For this review, take the finished solid that the model builds, in its own axes (mm). Face numbers are marked on the shaded views. A direction names the side the tool comes from. Coordinates: 2 decimals unless noted, no trailing zeros. Order: outer loops, then holes, each group sorted by start corner. A loop starts at its lowest first (then second) coordinate and runs counter-clockwise, first axis right, second up.
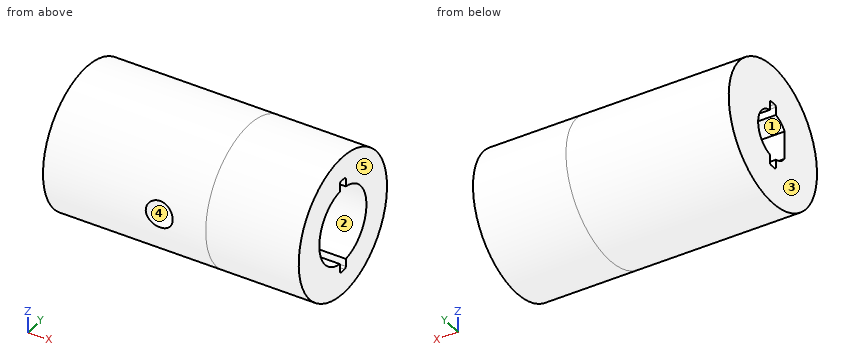
from build123d import *

# Parameters (mm, degrees)
SKETCH1_R            = 7.5
SKETCH1_R_2          = 4
SCREWSIDE_DEPTH      = 10
MOTORSIDE_START      = 17.5
SKETCH4_R            = 7.5
MOTORSIDE_DEPTH      = 17.5
SKETCH6_W            = 7
SKETCH6_H            = 1
ESCAPE_HOLES_DEPTH   = 30.474565306
SKETCH7_W            = 10
SKETCH7_H            = 1
ESCAPE_HOLES_2_DEPTH = 10
FILLET1_R            = 0.2
CUT_EXTRUDE3_DEPTH   = 22.277922831


with BuildPart() as part:
    # Sketch1 → ScrewSide (new body)
    with BuildSketch(Plane(origin=(0, 0, 0), x_dir=(0, 0, -1), z_dir=(1, 0, 0))):
        Circle(SKETCH1_R)
        Circle(SKETCH1_R_2, mode=Mode.SUBTRACT)
    extrude(amount=SCREWSIDE_DEPTH)

    # Sketch4 → MotorSide (add)
    with BuildSketch(Plane.ZY.offset(MOTORSIDE_START)):
        Circle(SKETCH4_R)
        with BuildLine():
            Line((-1.5, -2), (1.5, -2))
            ThreePointArc((1.5, -2), (0, 2.5), (-1.5, -2))
        make_face(mode=Mode.SUBTRACT)
    extrude(amount=-MOTORSIDE_DEPTH)

    # Sketch6 → Escape Holes (cut, through all)
    with BuildSketch(Plane.ZY.offset(17.5)):
        Rectangle(SKETCH6_W, SKETCH6_H)
    extrude(amount=-ESCAPE_HOLES_DEPTH, mode=Mode.SUBTRACT)

    # Sketch7 → Escape Holes 2 (cut)
    with BuildSketch(Plane(origin=(10, 0, 0), x_dir=(0, 0, -1), z_dir=(1, 0, 0))):
        Rectangle(SKETCH7_W, SKETCH7_H)
    extrude(amount=-ESCAPE_HOLES_2_DEPTH, mode=Mode.SUBTRACT)

    # Fillet1
    fillet1_edges = [part.edges().sort_by_distance(p)[0] for p in [
        (-8.75, 0.5, 3.5),
        (-8.75, -0.5, 3.5),
        (-8.75, -0.5, -3.5),
        (-8.75, 0.5, -3.5),
        (5, 0.5, 5),
        (5, -0.5, 5),
        (5, -0.5, -5),
        (5, 0.5, -5),
    ]]
    fillet(fillet1_edges, radius=FILLET1_R)

    # Sketch8 → Cut-Extrude3 (cut, through all)
    with BuildSketch(Plane(origin=(0, -2, 0), x_dir=(1, 0, 0), z_dir=(0, 1, 0))):
        with BuildLine():
            ThreePointArc((-6.45, 0), (-5, -1.45), (-3.55, 0))
            Line((-3.55, 0), (-6.45, 0))
        make_face()
        with BuildLine():
            Line((-6.45, 0), (-3.55, 0))
            ThreePointArc((-3.55, 0), (-5, 1.45), (-6.45, 0))
        make_face()
    extrude(amount=-CUT_EXTRUDE3_DEPTH, mode=Mode.SUBTRACT)


solid = part.part
1. Clearance check with flat-ended pins moving along their axes: pin 1 Ø0.7 at (x, z) = (6.5, -4.5) entering from -Y; pin 2 Ø5 at (x, y) = (-2.5, -4.5) entering from -Z; pin 3 Ø0.9 at (x, z) = (-13, 3) entering from -Y. State where each tip first meets the part, or that it passes through.
Answer below:
pin 1: stops at y = -6.25
pin 2: stops at z = -7.23
pin 3: stops at y = -7.05
2. Take a section at B-B, the plane x = -11.75. Give the boundary of the cut face in (y, z).
Answer below:
outline: circle Ø15 at (0, 0); hole (-2, -1.5) arc R2.5 ccw to (-0.5, -2.45) - (-0.5, -3.3) arc R0.2 ccw to (-0.3, -3.5) - (0.3, -3.5) arc R0.2 ccw to (0.5, -3.3) - (0.5, -2.45) arc R2.5 ccw to (0.5, 2.45) - (0.5, 3.3) arc R0.2 ccw to (0.3, 3.5) - (-0.3, 3.5) arc R0.2 ccw to (-0.5, 3.3) - (-0.5, 2.45) arc R2.5 ccw to (-2, 1.5) - close
3. The part is to be moulded in two halves that separate along Z. For the marked faces 4 and 5, say which applies: +Z half, -Z half, draft (parallel to the pull), parting line (faces both ways), or undercut.
Answer below:
face 4: undercut
face 5: draft
4. To check wall thickness, follow L1, parallel to Z at x = -4.5, y = 0; L2, parallel to Y at x = -7, z = 2; L3, parallel to X at y = -4.05, z = 0. State the ranges of each line that lie inside material, in increasing order.
Answer below:
L1: z = -7.5 to -3.5, 3.5 to 7.5
L2: y = -7.23 to -1.5, 1.5 to 7.23
L3: x = -17.5 to -6.45, -3.55 to 10
5. Take a section at C-C, the plane z = 1. Give the boundary of the cut face in (x, y), plus the area to 3 significant figures.
Answer below:
outline: (-17.5, -7.43) - (-6.05, -7.43) - (-6.05, -2) - (-17.5, -2) - close; (-17.5, 2.29) - (0, 2.29) - (0, 3.87) - (10, 3.87) - (10, 7.43) - (-17.5, 7.43) - close; (-3.95, -7.43) - (10, -7.43) - (10, -3.87) - (0, -3.87) - (0, -2) - (-3.95, -2) - close
area: 245 mm2
6. Machinability: for the marked faces 1, 2 and 3, which of the approach directions +Z, -Z, +X, -X, +Y, -Y give a long, thin tool a straight path to every point of the face, cutting with its end or side? Answer none if there is none.
Answer below:
face 1: +X, -X
face 2: +X
face 3: +Z, -Z, -X, +Y, -Y
7. Take a section at A-A, the plane y = 0. Give the boundary of the cut face in (x, z).
Answer below:
outline: (-17.5, -7.5) - (10, -7.5) - (10, -5) - (0, -5) - (0, -3.5) - (-17.5, -3.5) - close; (-17.5, 3.5) - (0, 3.5) - (0, 5) - (10, 5) - (10, 7.5) - (-17.5, 7.5) - close
8. Take a section at D-D, the plane y = 3.5. Give the boundary of the cut face in (x, z), plus the area to 3 significant figures.
Answer below:
outline: (-17.5, -6.63) - (10, -6.63) - (10, -1.94) - (0, -1.94) - (0, 1.94) - (10, 1.94) - (10, 6.63) - (-17.5, 6.63) - close
area: 326 mm2
